Verification items for the finished model (mm, model axes). Face numbers are marked on the shaded views. A direction names the side the tool comes from. Give positions to 0.01 mm unless a question says otherwise; leave off trailing zeros. Order: outer loops, then holes, each group sorted by start corner. A loop starts at its lowest first (then second) coordinate and runs counter-clockwise, first axis right, second up. Notation, with made-up numbers: (49, 12.25) -> (88, 12.25) arc R31 cw to (88, 44.25) -> close; hole circle Ø1 at (-3.75, -5). An arc over 180 degrees is marked (long way). Return JSON: item names as keys, results as strings. Group by question number.
(1) Tool access check on the marked faces 4, 5 and 6. Record the directions out of +Z, -Z, +X, -X, +Y, -Y that give a thin tool (end or side, any length) a straight path to the whole face; none if there is none.
(2) Depth check by flat-ended pin: pin 1 Ø5 at (x, y) = (-11.26, -6.5) entering from +Z; pin 2 Ø1 at (x, z) = (-16.5, 14.5) entering from -Y; pin 3 Ø6 at (y, z) = (-11, 2.5) entering from -X. Enter the tip coordinate at first touch or a pass-through.
(3) Cross-section at A-A on x = 0. Enter the section's corners in (y, z) (3 decimals).
(4) Release check for a two-part mould opening along Y. For the marked faces 1, 2 and 3 record: pulls with the +Y half, pulls with the -Y half, needs draft (parallel to the pull), parting line crosses it, or undercut.
(5) Cross-section at B-B on y = 0. Enter the section's corners in (x, z), then the cut area to 3 significant figures.
(6) Cross-section at C-C on z = 14. Enter the section's corners in (x, y), then the cut area to 3 significant figures.
(7) Thickness scan on line 1 along Z through (x, y) = (-17, -16); line 2 along Y through (x, z) = (0, 13.25); line 3 along Y through (x, z) = (-11.5, 3.75). Record the ranges inside material, lowest first.
(8) Cross-section at D-D on y = 13. Enter the section's corners in (x, z) (3 decimals).
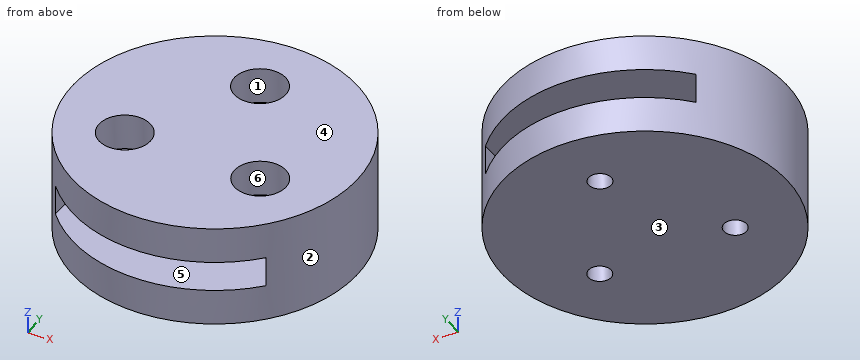
from build123d import *

# Parameters (mm, degrees)
F0_R     = 23.5
F1_DEPTH = 17
F2_W     = 35
F2_H     = 5
F3_DEPTH = 28.6
F4_R     = 1.875
F5_DEPTH = 17.001
F6_R     = 4.25
F7_DEPTH = 14.25
F8_SIZE  = 2


with BuildPart() as f1:
    # F0 (on Top) → F1 (new body)
    with BuildSketch(Plane.XY):
        Circle(F0_R)
    extrude(amount=F1_DEPTH)

    # F2 (on Front) → F3 (cut, symmetric)
    with BuildSketch(Plane.XZ):
        with Locations((0, 8.5)):
            Rectangle(F2_W, F2_H)
    extrude(amount=F3_DEPTH, both=True, mode=Mode.SUBTRACT)

    # F4 (on face) → F5 (cut, through all)
    with BuildSketch(Plane.XY.offset(17)):
        with Locations((0, 13)):
            Circle(F4_R)
        with Locations((-11.25833, -6.5)):
            Circle(F4_R)
        with Locations((11.25833, -6.5)):
            Circle(F4_R)
    extrude(amount=-F5_DEPTH, mode=Mode.SUBTRACT)

    # F6 (on face) → F7 (cut)
    with BuildSketch(Plane.XY.offset(17)):
        with Locations((0, 13)):
            Circle(F6_R)
        with Locations((-11.25833, -6.5)):
            Circle(F6_R)
        with Locations((11.25833, -6.5)):
            Circle(F6_R)
    extrude(amount=-F7_DEPTH, mode=Mode.SUBTRACT)

    # F8
    f8_edges = [f1.edges().sort_by_distance(p)[0] for p in [
        (-15.50833, -6.5, 2.75),
        (7.00833, -6.5, 2.75),
        (-4.25, 13, 2.75),
    ]]
    chamfer(f8_edges, length=F8_SIZE)


solid = f1.part
Verdict:
{
 "1": {"face 4": "+Z, +X, -X, +Y, -Y", "face 5": "+Y, -Y", "face 6": "+Z"},
 "2": {"pin 1": "z = 3", "pin 2": "y = -17.21", "pin 3": "x = -22.1"},
 "3": {"outline": "(-23.5, 0) -> (11.125, 0) -> (11.125, 2.75) -> (10.75, 2.75) -> (8.75, 4.75) -> (8.75, 6) -> (-23.5, 6) -> close; (-23.5, 11) -> (8.75, 11) -> (8.75, 17) -> (-23.5, 17) -> close; (14.875, 0) -> (23.5, 0) -> (23.5, 6) -> (17.25, 6) -> (17.25, 4.75) -> (15.25, 2.75) -> (14.875, 2.75) -> close; (17.25, 11) -> (23.5, 11) -> (23.5, 17) -> (17.25, 17) -> close"},
 "4": {"face 1": "undercut", "face 2": "parting line crosses it", "face 3": "needs draft"},
 "5": {"outline": "(-23.5, 0) -> (23.5, 0) -> (23.5, 17) -> (-23.5, 17) -> close; hole (-17.5, 6) -> (17.5, 6) -> (17.5, 11) -> (-17.5, 11) -> close", "area": "624 mm²"},
 "6": {"outline": "circle Ø47 at (0, 0); hole circle Ø8.5 at (-11.26, -6.5); hole circle Ø8.5 at (0, 13); hole circle Ø8.5 at (11.26, -6.5)", "area": "1,560 mm²"},
 "7": {"line 1": "0 to 6, 11 to 17", "line 2": "-23.5 to 8.75, 17.25 to 23.5", "line 3": "-20.49 to -9.74, -3.26 to 20.49"},
 "8": {"outline": "(-19.577, 0) -> (-1.875, 0) -> (-1.875, 2.75) -> (-2.25, 2.75) -> (-4.25, 4.75) -> (-4.25, 6) -> (-17.5, 6) -> (-17.5, 11) -> (-4.25, 11) -> (-4.25, 17) -> (-19.577, 17) -> close; (1.875, 0) -> (19.577, 0) -> (19.577, 17) -> (4.25, 17) -> (4.25, 11) -> (17.5, 11) -> (17.5, 6) -> (4.25, 6) -> (4.25, 4.75) -> (2.25, 2.75) -> (1.875, 2.75) -> close"}
}
